Check sheet for the drawn part. Datum: minimum x, y, z corner. Units: mm. A direction names the side the tool comes from. Coordinates: 2 decimals unless noted, no trailing zeros. Loops run counter-clockwise (first coordinate to the right, second up) from the corner with the lowest first, then second, coordinate; pieces in that order, holes last.
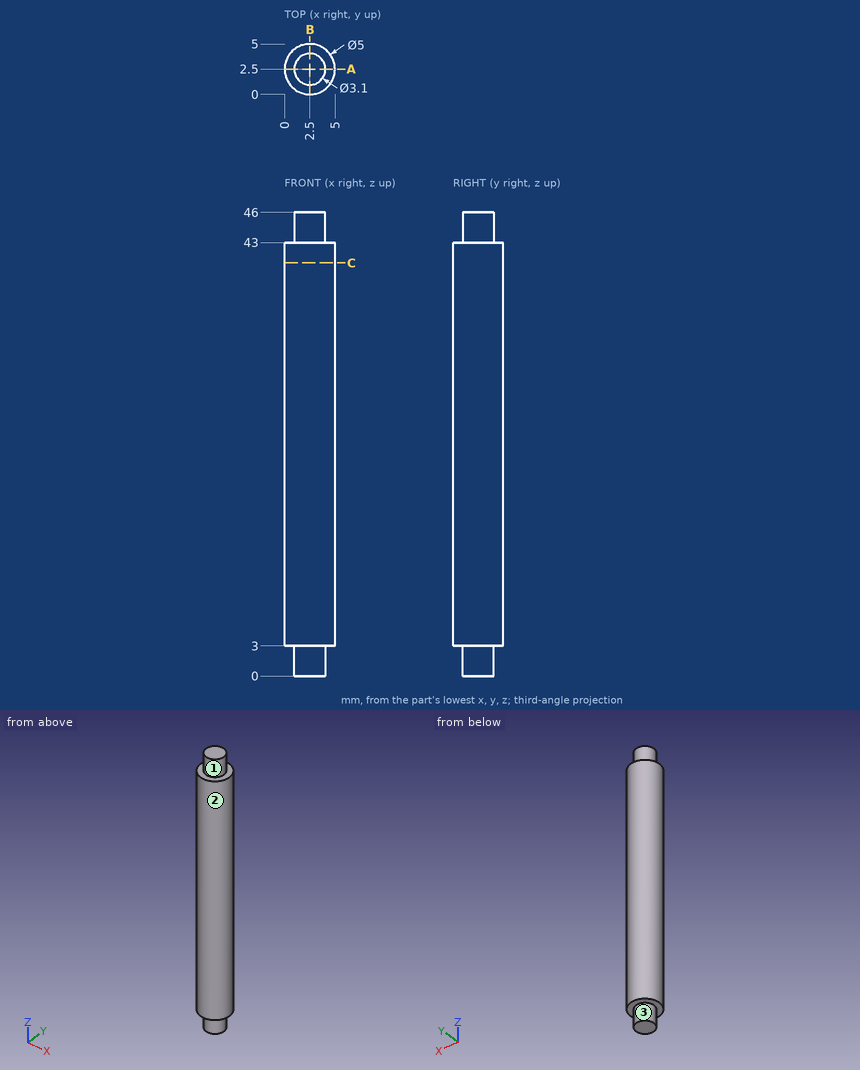
1) Scan lines: line 1 (Y direction, x = 2.65, z = 30); line 2 (Z direction, x = 4, y = 4); line 3 (Y direction, x = 3.3, z = 19.5). Record each from-to range of solid material in increasing order.
Answer sheet:
line 1: y = 0 to 5
line 2: z = 3 to 43
line 3: y = 0.13 to 4.87
2) Set-up check for the marked faces 1, 2 and 3: record each of +Z, -Z, +X, -X, +Y, -Y from which the full face is reachable in a straight line by a thin tool's end or side.
Answer sheet:
face 1: +Z
face 2: +Z, -Z
face 3: -Z
3) Section check C-C on z = 41. Enter the section's corners in (x, y).
Answer sheet:
outline: circle Ø5 at (2.5, 2.5)
4) Depth check by flat-ended pin: pin 1 (1.5 mm diameter, centred on y = 1, z = 11, fed in from -X); pin 2 (2 mm diameter, centred on y = 1, z = 25, fed in from +X); pin 3 (1.5 mm diameter, centred on x = 4.5, z = 21, fed in from +Y). Enter the tip coordinate at first touch or a pass-through.
Answer sheet:
pin 1: stops at x = 0.12
pin 2: stops at x = 4.95
pin 3: stops at y = 4.67
5) Section check A-A on y = 2.5. Enter the section's corners in (x, z), plus the area to 3 significant figures.
Answer sheet:
outline: (0, 3) - (0.95, 3) - (0.95, 0) - (4.05, 0) - (4.05, 3) - (5, 3) - (5, 43) - (4.05, 43) - (4.05, 46) - (0.95, 46) - (0.95, 43) - (0, 43) - close
area: 219 mm2
